```python
from build123d import *

# Parameters (mm, degrees)
SKETCH1_W           = 100
SKETCH1_H           = 100
BOSS_EXTRUDE1_DEPTH = 100
SHELL1_T            = -5
BOSS_EXTRUDE2_REACH = 214.132
SKETCH2_W           = 5
SKETCH2_H           = 10


with BuildPart() as part:
    # Sketch1 → Boss-Extrude1 (new, symmetric)
    with BuildSketch(Plane(origin=(0, 0, 0), x_dir=(-1, 0, 0), z_dir=(0, 1, 0))):
        Rectangle(SKETCH1_W, SKETCH1_H)
    extrude(amount=BOSS_EXTRUDE1_DEPTH, both=True)

    # Shell1
    shell1_openings = [part.faces().sort_by_distance(p)[0] for p in [
        (0, 100, 0),
    ]]
    offset(amount=SHELL1_T, openings=shell1_openings, kind=Kind.INTERSECTION)

    # Sketch2 → Boss-Extrude2 (add, up to next)
    with BuildSketch(Plane(origin=(0, 100, 0), x_dir=(-1, 0, 0), z_dir=(0, 1, 0)), mode=Mode.PRIVATE) as boss_extrude2_sk1:
        with Locations((-42.5, -40)):
            Rectangle(SKETCH2_W, SKETCH2_H)
    boss_extrude2_tool1 = extrude(boss_extrude2_sk1.sketch, amount=-BOSS_EXTRUDE2_REACH, mode=Mode.PRIVATE) - part.part
    # Sketch2 → Boss-Extrude2 (add, up to next)
    with BuildSketch(Plane(origin=(0, 100, 0), x_dir=(-1, 0, 0), z_dir=(0, 1, 0)), mode=Mode.PRIVATE) as boss_extrude2_sk2:
        with Locations((42.5, -40)):
            Rectangle(SKETCH2_W, SKETCH2_H)
    boss_extrude2_tool2 = extrude(boss_extrude2_sk2.sketch, amount=-BOSS_EXTRUDE2_REACH, mode=Mode.PRIVATE) - part.part
    add(boss_extrude2_tool1.solids().sort_by_distance((42.5, 100, -40))[0])
    add(boss_extrude2_tool2.solids().sort_by_distance((-42.5, 100, -40))[0])


solid = part.part
```
Read the model definition and answer for the solid it produces. Units are mm, in the model's axes. A direction names the side the tool comes from. Give positions to 0.01 mm unless a question says otherwise; leave off trailing zeros. Write each loop counter-clockwise with the first axis right and the second up, starting at its lowest first coordinate (ties: lowest second). Pieces come first, ordered by that corner, then holes. Notation, with made-up numbers: (85, 13) - (94, 13) arc R31 ccw to (94, 51) - close; hole circle Ø6 at (84.5, 79). An arc over 180 degrees is marked (long way). Write item = value, one per line. Start each with the question number.
Item 1: Find the intervals of material crossed by probe 1 along Z at (x, y) = (25.5, 23.5); probe 2 along Y at (x, z) = (18, 26.5), in increasing order. Write a range as [from, to].
Item 2: A tool of negligible diameter and unlimited length cuts with its end or side. For faces 1 (the flat face through (-50, 1, -1)), 2 (the flat face through (-40, 4, -40)), from which of +Z, -Z, +X, -X, +Y, -Y can it reach the whole face along a straight path? Write none if from no direction.
Item 3: The mould has two halves that part along Z. Classify faces 3 (the flat face through (45, 4, 4)), 4 (the flat face through (1, 1, -50)), 5 (the flat face through (1, 1, 50)): +Z half, -Z half, draft (parallel to the pull), parting line (faces both ways), or undercut.
Item 4: Find section A-A (y = -67). Give the vertices of the cut face in (x, z), then the cut area to 3 significant figures.
Item 5: Find section B-B (x = 34). Give the vertices of the cut face in (y, z), then the cut area to 3 significant figures.
Item 6: This flat-tipped pin is pushed along its axis until it touches: P1, Ø12, axis at x = -23, z = 31, coming from the +Y side. Where does it stop, or does it pass through?
Item 7: Find section C-C (z = -4.5). Give the vertices of the cut face in (x, y).
Response:
q1.probe_1 = [-50, -45], [45, 50]
q1.probe_2 = [-100, -95]
q2.face_1 = +Z, -Z, -X, +Y, -Y
q2.face_2 = +Y
q3.face_3 = undercut
q3.face_4 = -Z half
q3.face_5 = +Z half
q4.outline = (-50, -50) - (50, -50) - (50, 50) - (-50, 50) - close; hole (-45, -35) - (-40, -35) - (-40, -45) - (40, -45) - (40, -35) - (45, -35) - (45, 45) - (-45, 45) - close
q4.area = 2,000 mm²
q5.outline = (-100, -50) - (100, -50) - (100, -45) - (-95, -45) - (-95, 45) - (100, 45) - (100, 50) - (-100, 50) - close
q5.area = 2,450 mm²
q6.P1 = -95
q7.outline = (-50, -100) - (50, -100) - (50, 100) - (45, 100) - (45, -95) - (-45, -95) - (-45, 100) - (-50, 100) - close
